```python
from build123d import *

# Parameters (mm, degrees)
SKETCH1_W           = 40
SKETCH1_H           = 40
BOSS_EXTRUDE1_DEPTH = 50
FILLET1_R           = 6
SKETCH2_R           = 15.025
CUT_EXTRUDE1_DEPTH  = 50


with BuildPart() as part:
    # Sketch1 → Boss-Extrude1 (new body)
    with BuildSketch(Plane.XY):
        Rectangle(SKETCH1_W, SKETCH1_H)
    extrude(amount=BOSS_EXTRUDE1_DEPTH)

    # Fillet1
    fillet1_edges = [part.edges().sort_by_distance(p)[0] for p in [
        (-20, 0, 50),
        (0, -20, 50),
        (20, 0, 50),
        (0, -20, 0),
        (-20, 0, 0),
        (0, 20, 0),
        (20, 0, 0),
        (0, 20, 50),
        (20, -20, 25),
        (-20, -20, 25),
        (-20, 20, 25),
        (20, 20, 25),
    ]]
    fillet(fillet1_edges, radius=FILLET1_R)

    # Sketch2 → Cut-Extrude1 (cut)
    with BuildSketch(Plane(origin=(0, 20, 0), x_dir=(1, 0, 0), z_dir=(0, 1, 0))):
        with Locations(Location((0, -25, 0), (0, 0, 201.285935721))):
            Circle(SKETCH2_R)
    extrude(amount=-CUT_EXTRUDE1_DEPTH, mode=Mode.SUBTRACT)


solid = part.part
```
Check sheet for the modelled part. Datum: model origin and axes. Units: mm. Round coordinates to 2 decimals unless told otherwise and drop trailing zeros. Order: outer loops, then holes, each group sorted by start corner. A loop starts at its lowest first (then second) coordinate and runs counter-clockwise, first axis right, second up. Notation, with made-up numbers: M 49,62.25 L 83,62.25 A21 ccw 83,98.25 Z; hole C 64,26 d9. An arc over 180 degrees is marked long. Answer in a Markdown table with one row per item.
(1) Material ranges on line 1 along X through (y, z) = (-7, 25) (3 decimals); line 2 along Z through (x, y) = (0, -8) (3 decimals); line 3 along Z through (x, y) = (10.5, 9), recorded low to high. Write a range as from..to.
Findings:
| item | result |
|---|---|
| line 1 | x = -20..-15.025, 15.025..20 |
| line 2 | z = 0..9.975, 40.025..50 |
| line 3 | z = 0..14.25, 35.75..50 |
(2) Draft check along Z on faces 1 (the cylindrical face through (-18.289, -18.196, 25.266)), 2 (the cylindrical face through (-18.289, 0.196, 1.804)), 3 (the cylindrical face through (-15.02, 0.28, 24.68)). Enter one of: +Z half, -Z half, draft (parallel to the pull), parting line (faces both ways), or undercut.
Findings:
| item | result |
|---|---|
| face 1 | draft |
| face 2 | -Z half |
| face 3 | undercut |
(3) Section check B-B on x = 0. Record the boundary of the cut face in (y, z) (3 decimals).
Findings:
| item | result |
|---|---|
| outline | M -20,6 A6 ccw -14,0 L 14,0 A6 ccw 20,6 L 20,9.975 L -20,9.975 Z; M -20,40.025 L 20,40.025 L 20,44 A6 ccw 14,50 L -14,50 A6 ccw -20,44 Z |
(4) Section check A-A on y = -9.5. Record the boundary of the cut face in (x, z) (3 decimals), plus the area to 3 significant figures.
Findings:
| item | result |
|---|---|
| outline | M -20,6 A6 ccw -14,0 L 14,0 A6 ccw 20,6 L 20,44 A6 ccw 14,50 L -14,50 A6 ccw -20,44 Z; hole C 0,25 d30.05 |
| area | 1,260 mm^2 |
(5) Gauge pin test, flat ends, axial feed: pin 1 (18 mm diameter, centred on x = 0, z = 25, fed in from -Y); pin 2 (2 mm diameter, centred on x = -15, z = 44.5, fed in from -Y). Record the tip position at first contact, or that the pin passes through.
Findings:
| item | result |
|---|---|
| pin 1 | passes through |
| pin 2 | stops at y = -20 |
(6) Section check D-D on z = 8. Record the boundary of the cut face in (x, y).
Findings:
| item | result |
|---|---|
| outline | M -20,-14 A6 ccw -14,-20 L 14,-20 A6 ccw 20,-14 L 20,14 A6 ccw 14,20 L -14,20 A6 ccw -20,14 Z |
(7) Section check C-C on z = 25. Record the boundary of the cut face in (x, y) (3 decimals), plus the area to 3 significant figures.
Findings:
| item | result |
|---|---|
| outline | M -20,-14 A6 ccw -15.025,-19.912 L -15.025,19.912 A6 ccw -20,14 Z; M 15.025,-19.912 A6 ccw 20,-14 L 20,14 A6 ccw 15.025,19.912 Z |
| area | 367 mm^2 |
